Here's how the part is built. I have some questions about the finished solid (model axes, mm). Face numbers are marked on the shaded views. A direction names the side the tool comes from. Round coordinates to 2 decimals unless told otherwise and drop trailing zeros. Order: outer loops, then holes, each group sorted by start corner. A loop starts at its lowest first (then second) coordinate and runs counter-clockwise, first axis right, second up.
```python
from build123d import *

# Parameters (mm, degrees)
F0_R     = 14.5
F0_R_2   = 9.3
F1_DEPTH = 8
F2_DEPTH = 12.5
F0_R_3   = 6
F3_DEPTH = 6.6
F4_DEPTH = 5.9
F5_DEPTH = 5.9


with BuildPart() as f1:
    # F0 (on Top) → F1 (new body, symmetric)
    with BuildSketch(Plane.XY):
        with BuildLine():
            Line((2.6379834818, -18.8137083294), (11.6484677091, -17.5502940073))
            Line((11.6484677091, -17.5502940073), (37.9808631577, 38.9197102657))
            Line((37.9808631577, 38.9197102657), (16.6523997132, 89.1664213307))
            ThreePointArc((16.6523997132, 89.1664213307), (12.1489449291, 89.292756528), (7.6523997132, 89.0132092222))
            ThreePointArc((7.6523997132, 89.0132092222), (3.6651197911, 48.1806616582), (-15.0070128486, 11.6492121327))
            ThreePointArc((-15.0070128486, 11.6492121327), (-16.4391484767, -9.5220257988), (2.6379834818, -18.8137083294))
        make_face()
        Circle(F0_R, mode=Mode.SUBTRACT)
        with Locations((21.8, 31.3)):
            Circle(F0_R_2, mode=Mode.SUBTRACT)
    extrude(amount=F1_DEPTH, both=True)

    # F0 (on Top) → F2 (join, symmetric)
    with BuildSketch(Plane.XY):
        with BuildLine():
            Line((11.6484677091, -17.5502940073), (49.9478345026, -12.1801088639))
            ThreePointArc((49.9478345026, -12.1801088639), (61.4641714079, 8.1340479446), (80.9495714617, 21.0030093362))
            ThreePointArc((80.9495714617, 21.0030093362), (77.7070823253, 27.4172128648), (71, 30))
            Line((71, 30), (48.3859111453, 30))
            ThreePointArc((48.3859111453, 30), (42.8665412922, 31.6611417793), (39.1808626108, 36.0926887151))
            Line((39.1808626108, 36.0926887151), (37.9808631577, 38.9197102657))
            Line((37.9808631577, 38.9197102657), (11.6484677091, -17.5502940073))
        make_face()
    extrude(amount=F2_DEPTH, both=True)



with BuildPart() as f3:
    # F0 (on Top) → F3 (new body, symmetric)
    with BuildSketch(Plane.XY):
        with BuildLine():
            Line((49.9478345026, -12.1801088639), (73.2497189898, -8.9128111416))
            ThreePointArc((73.2497189898, -8.9128111416), (78.7914457558, -5.9056129695), (81, 0))
            Line((81, 0), (81, 20))
            ThreePointArc((81, 20), (80.9873849084, 20.5021381199), (80.9495714617, 21.0030093362))
            ThreePointArc((80.9495714617, 21.0030093362), (61.4641714079, 8.1340479446), (49.9478345026, -12.1801088639))
        make_face()
        with Locations((72, 0)):
            Circle(F0_R_3, mode=Mode.SUBTRACT)
    extrude(amount=F3_DEPTH, both=True)


with BuildPart() as f1_1:
    add(f1.part)
    # F4 (add, through all): a face of the model
    f4_faces = [f3.part.faces().sort_by_distance(p)[0] for p in [
        (61.7962542599, 7.8237954492, 6.6),
    ]]
    extrude(f4_faces, amount=F4_DEPTH)

    # F5 (add, through all): a face of the model
    f5_faces = [f3.part.faces().sort_by_distance(p)[0] for p in [
        (61.7962542599, 7.8237954492, -6.6),
    ]]
    extrude(f5_faces, amount=F5_DEPTH)

    # F6: cut F3
    add(f3.part, mode=Mode.SUBTRACT)


solid = f1_1.part
```
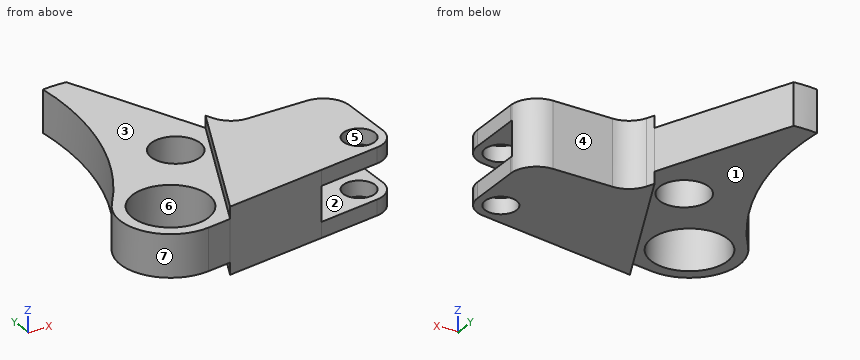
1. If we section it at D-D, the plane y = -3.5: Write out the boundary of the cut face in (x, z), and give its area (3 significant figures).
Evaluation:
outline: (-18.67, -8) - (-14.07, -8) - (-14.07, 8) - (-18.67, 8) - close; (14.07, -8) - (18.2, -8) - (18.2, -12.5) - (67.13, -12.5) - (67.13, -6.6) - (53.35, -6.6) - (53.35, 6.6) - (67.13, 6.6) - (67.13, 12.5) - (18.2, 12.5) - (18.2, 8) - (14.07, 8) - close; (76.87, -12.5) - (80.29, -12.5) - (80.29, -6.6) - (76.87, -6.6) - close; (76.87, 6.6) - (80.29, 6.6) - (80.29, 12.5) - (76.87, 12.5) - close
area: 1,220 mm2
2. If we section it at C-C, the plane z = 9.75: Write out the boundary of the cut face in (x, y).
Evaluation:
outline: (11.65, -17.55) - (73.25, -8.91) arc R9 ccw to (81, 0) - (81, 20) arc R10 ccw to (71, 30) - (48.39, 30) arc R10 cw to (39.18, 36.09) - (37.98, 38.92) - close; hole circle Ø12 at (72, 0)
3. If we mould it in two halves opening along Y, with no side actions, what happens to the marked faces 4, 5, 6 and 7? For each: released by +Y, released by -Y, zero draft, split by the parting line, or undercut.
Evaluation:
face 4: released by +Y
face 5: undercut
face 6: undercut
face 7: split by the parting line
4. I'm going to push flat-ended pins straight in: P1, Ø17, axis at x = 0, y = 12, coming from the -Z side; P2, Ø2, axis at x = 16.5, z = 0, coming from the +Y side; P3, Ø1, axis at y = 26, z = -2, coming from the -X side. Where does each tip first touch, or does it pass through?
Evaluation:
P1: stops at z = -8
P2: stops at y = 89.24
P3: stops at x = -5.84
5. If we section it at B-B, the plane x = 21.8: Write out the boundary of the cut face in (y, z).
Evaluation:
outline: (-16.13, -12.5) - (4.22, -12.5) - (4.22, -8) - (22, -8) - (22, 8) - (4.22, 8) - (4.22, 12.5) - (-16.13, 12.5) - close; (40.6, -8) - (77.04, -8) - (77.04, 8) - (40.6, 8) - close
6. On a 3-axis mill with a long thin cutter (end or side, diameter ignored), from which of +Z, -Z, +X, -X, +Y, -Y can I reach the whole of each face in a straight line? I mean the marked faces 1, 2 and 3. Say none if no direction works.
Evaluation:
face 1: -Z, -X, +Y
face 2: +X, -Y
face 3: +Z, -X, +Y
7. If we section it at A-A, the plane z = -3.75: Write out the boundary of the cut face in (x, y), and give its area (3 significant figures).
Evaluation:
outline: (-15.01, 11.65) arc R19 ccw to (2.64, -18.81) - (49.95, -12.18) arc R50 cw to (80.95, 21) arc R10 ccw to (71, 30) - (48.39, 30) arc R10 cw to (39.18, 36.09) - (16.65, 89.17) arc R50 ccw to (7.65, 89.01) arc R110 cw to start; hole circle Ø29 at (0, 0); hole circle Ø18.6 at (21.8, 31.3)
area: 4,050 mm2
8. I need wall thicknesses on probe 1 along Z at (x, y) = (3, 28); probe 2 along Y at (x, z) = (72, -9.1); probe 3 along Y at (x, z) = (10.5, -6.75). Which ranges of each line are inside material? Lowest first, please.
Evaluation:
probe 1: z = -8 to 8
probe 2: y = -9.09 to -6, 6 to 29.95
probe 3: y = -17.71 to -10, 10 to 89.24
